from build123d import *

# Parameters (mm, degrees)
F0_R     = 2.5
F1_DEPTH = 3.75


with BuildPart() as f1:
    # F0 (on Top) → F1 (new body, symmetric)
    with BuildSketch(Plane.XY):
        with BuildLine():
            ThreePointArc((53.8125, -1.210307), (53.5, 0), (53.8125, 1.210307))
            ThreePointArc((53.8125, 1.210307), (52.362072, 3.228098), (50, 4))
            Line((50, 4), (0, 4))
            ThreePointArc((0, 4), (-4, 0), (0, -4))
            Line((0, -4), (50, -4))
            ThreePointArc((50, -4), (52.362072, -3.228098), (53.8125, -1.210307))
        make_face()
        Circle(F0_R, mode=Mode.SUBTRACT)
        with Locations((8, 0)):
            Circle(F0_R, mode=Mode.SUBTRACT)
        with Locations((16, 0)):
            Circle(F0_R, mode=Mode.SUBTRACT)
        with Locations((24, 0)):
            Circle(F0_R, mode=Mode.SUBTRACT)
        with Locations((32, 0)):
            Circle(F0_R, mode=Mode.SUBTRACT)
        with Locations((40, 0)):
            Circle(F0_R, mode=Mode.SUBTRACT)
        with Locations((48, 0)):
            Circle(F0_R, mode=Mode.SUBTRACT)
    extrude(amount=F1_DEPTH, both=True)


solid = f1.part
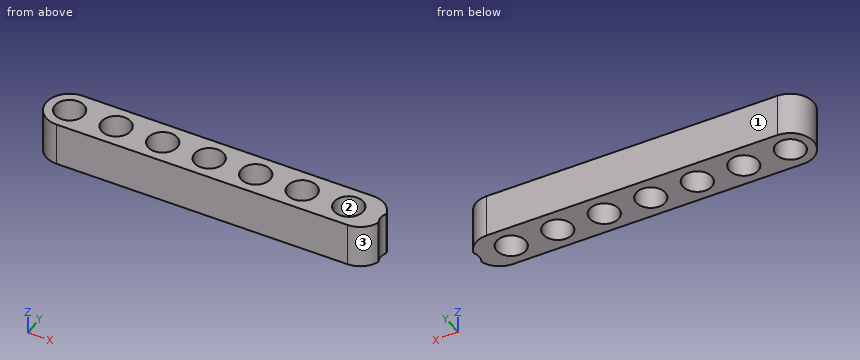
Can you work these out from the model? Positions are in its coordinate system, mm. Face numbers are marked on the shaded views. Give positions to 0.01 mm unless a question says otherwise; leave off trailing zeros. Write each loop counter-clockwise with the first axis right and the second up, starting at its lowest first coordinate (ties: lowest second). Pieces come first, ordered by that corner, then holes. Notation, with made-up numbers: (35, 30) -> (94, 30) arc R20 cw to (94, 68) -> close; hole circle Ø5 at (-34.75, 78). An arc over 180 degrees is marked (long way). Answer as a JSON object with one key per item and string values. Group by question number.
Item 1: I'm going to push flat-ended pins straight in: P1, Ø3, axis at x = 16, y = 0, coming from the +Z side; P2, Ø1, axis at y = -1.5, z = 1.5, coming from the -X side; P3, Ø1, axis at y = 0, z = 2.5, coming from the +X side. Where does each tip first touch, or does it pass through?
Item 2: Suppose I cut it at B-B (y = 0). State how many separate pieces and enclosed holes the cut face has, plus the area to 3 significant figures.
Item 3: Suppose I cut it at A-A (x = 2). Please give me the cut outline in (y, z), plus the area to 3 significant figures.
Item 4: Suppose I cut it at C-C (z = -2.5). Please give me the cut outline in (x, y), plus the area to 3 significant figures.
Item 5: We'd pull the mould along Y, two halves only. Please class the marked faces 1, 2 and 3: +Y half, -Y half, draft (parallel to the pull), parting line (faces both ways), or undercut.
Item 6: Suppose I cut it at D-D (x = 40). Please give me the cut outline in (y, z), plus the area to 3 significant figures.
Item 7: Please list where these lines run through material, in increasing order: line 1 (Y direction, x = 48, z = 2); line 2 (Y direction, x = 0.5, z = 0.5); line 3 (X direction, y = 3, z = 1.25). Write a range as [from, to].
Findings:
{
 "1": {"P1": "passes through", "P2": "stops at x = -3.87", "P3": "stops at x = 53.55"},
 "2": {"separate pieces": "8", "enclosed holes": "0", "area": "169 mm²"},
 "3": {"outline": "(-4, -3.75) -> (-1.5, -3.75) -> (-1.5, 3.75) -> (-4, 3.75) -> close; (1.5, -3.75) -> (4, -3.75) -> (4, 3.75) -> (1.5, 3.75) -> close", "area": "37.5 mm²"},
 "4": {"outline": "(0, -4) -> (50, -4) arc R4 ccw to (53.81, -1.21) arc R2.5 cw to (53.81, 1.21) arc R4 ccw to (50, 4) -> (0, 4) arc R4 ccw to start; hole circle Ø5 at (0, 0); hole circle Ø5 at (8, 0); hole circle Ø5 at (16, 0); hole circle Ø5 at (24, 0); hole circle Ø5 at (32, 0); hole circle Ø5 at (40, 0); hole circle Ø5 at (48, 0)", "area": "312 mm²"},
 "5": {"face 1": "+Y half", "face 2": "undercut", "face 3": "-Y half"},
 "6": {"outline": "(-4, -3.75) -> (-2.5, -3.75) -> (-2.5, 3.75) -> (-4, 3.75) -> close; (2.5, -3.75) -> (4, -3.75) -> (4, 3.75) -> (2.5, 3.75) -> close", "area": "22.5 mm²"},
 "7": {"line 1": "y = [-4, -2.5], [2.5, 4]", "line 2": "y = [-4, -2.45], [2.45, 4]", "line 3": "x = [-2.65, 52.65]"}
}
